For this review, use the dimensioned drawing (mm, ordinates from the lowest corner) and the shaded views. A direction names the side the tool comes from. Round coordinates to 2 decimals unless told otherwise and drop trailing zeros. Write each loop counter-clockwise with the first axis right and the second up, starting at its lowest first coordinate (ties: lowest second). Pieces come first, ordered by that corner, then holes.
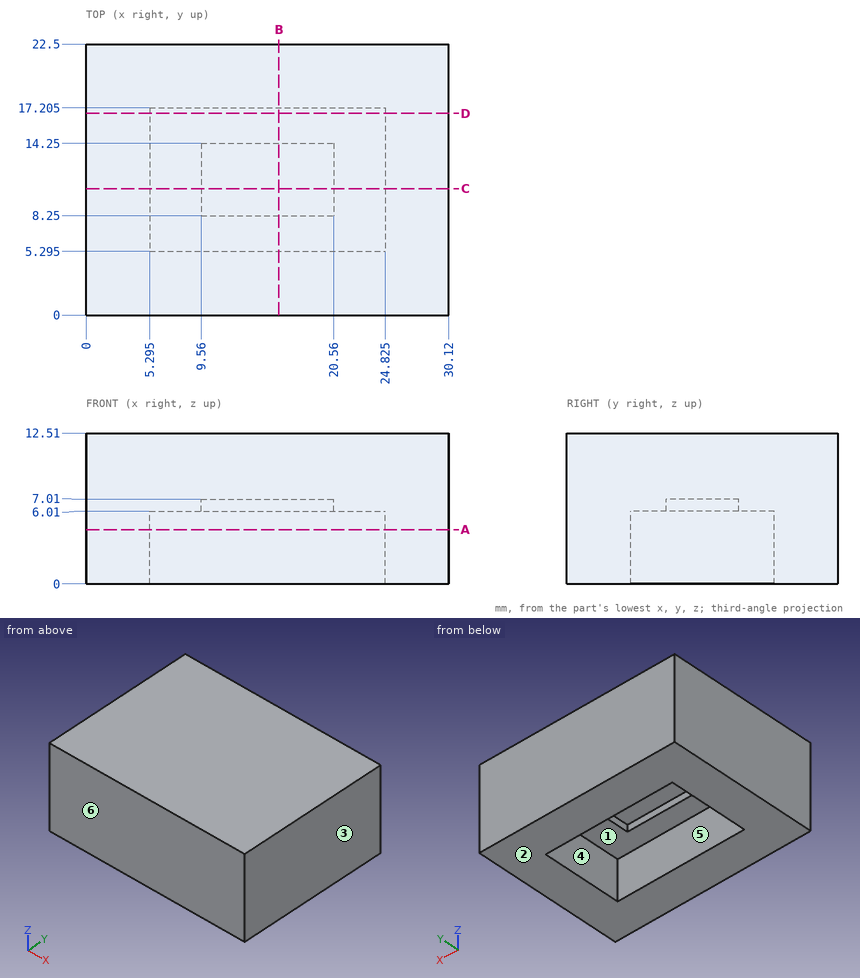
1) For line 1 along X through (y, z) = (10.5, 2.75) (3 decimals); line 2 along Y through (x, z) = (9.5, 5.5) (3 decimals); line 3 along Z through (x, y) = (11, 5.75), list the stretches that pass through material, from the lowest coordinate up.
2) Add section A-A on z = 4.5. State the section outline as (x, y) points (3 decimals), and give its area (3 significant figures).
3) For P1, Ø3, axis at x = 13, y = 14, coming from the -Z side, flat-tipped, find the tip position at first contact; note if it passes through.
4) For the marked faces 5 and 6, list the 3-axis set-ups (+Z, -Z, +X, -X, +Y, -Y) from which the entire face can be reached by the end or side of a thin tool; tool diameter is ignored.
5) Add section C-C on y = 10.5. State the section outline as (x, z) points (3 decimals).
6) Add section D-D on y = 16.75. State the section outline as (x, z) points (3 decimals), and give its area (3 significant figures).
7) The part is to be moulded in two halves that separate along X. For the marked faces 1, 2, 3 and 4, say which applies: pulls with the +X half, pulls with the -X half, needs draft (parallel to the pull), parting line crosses it, or undercut.
8) Add section B-B on x = 16. State the section outline as (y, z) points (3 decimals), and give its area (3 significant figures).
Computed:
1. line 1: x = 0 to 5.295, 24.825 to 30.12
1. line 2: y = 0 to 5.295, 17.205 to 22.5
1. line 3: z = 6.01 to 12.51
2. outline: (0, 0) - (30.12, 0) - (30.12, 22.5) - (0, 22.5) - close; hole (5.295, 5.295) - (24.825, 5.295) - (24.825, 17.205) - (5.295, 17.205) - close
2. area: 445 mm2
3. P1: stops at z = 6.01
4. face 5: -Z
4. face 6: +Z, -Z, +X, -X, -Y
5. outline: (0, 0) - (5.295, 0) - (5.295, 6.01) - (9.56, 6.01) - (9.56, 7.01) - (20.56, 7.01) - (20.56, 6.01) - (24.825, 6.01) - (24.825, 0) - (30.12, 0) - (30.12, 12.51) - (0, 12.51) - close
6. outline: (0, 0) - (5.295, 0) - (5.295, 6.01) - (24.825, 6.01) - (24.825, 0) - (30.12, 0) - (30.12, 12.51) - (0, 12.51) - close
6. area: 259 mm2
7. face 1: undercut
7. face 2: needs draft
7. face 3: pulls with the +X half
7. face 4: undercut
8. outline: (0, 0) - (5.295, 0) - (5.295, 6.01) - (8.25, 6.01) - (8.25, 7.01) - (14.25, 7.01) - (14.25, 6.01) - (17.205, 6.01) - (17.205, 0) - (22.5, 0) - (22.5, 12.51) - (0, 12.51) - close
8. area: 204 mm2
